The model under review builds one solid part; all positions refer to its coordinate system, in mm. A direction names the side the tool comes from. Coordinates: 2 decimals unless noted, no trailing zeros. Loops run counter-clockwise (first coordinate to the right, second up) from the corner with the lowest first, then second, coordinate; pieces in that order, holes last. Notation, with made-up numbers: M 29,-20 L 81,-20 A21 ccw 81,9 Z; hole C 74.5,48.25 d8. An arc over 180 degrees is marked long. Return JSON: item names as keys, results as strings.
```python
from build123d import *

# Parameters (mm, degrees)
SKETCH1_R           = 2.637642313
SKETCH1_R_2         = 73
BOSS_EXTRUDE1_DEPTH = 20
SKETCH7_R           = 73
SKETCH7_R_2         = 52.25
BOSS_EXTRUDE2_DEPTH = 10
SKETCH8_R           = 73
BOSS_EXTRUDE3_DEPTH = 10
SKETCH9_R           = 11.25
CUT_EXTRUDE1_DEPTH  = 3
SKETCH10_R          = 4.5
CUT_EXTRUDE2_DEPTH  = 89
SKETCH11_R          = 55.2
SKETCH11_R_2        = 52.25
CUT_EXTRUDE3_DEPTH  = 10
SKETCH12_R          = 1
CUT_EXTRUDE4_DEPTH  = 224
SKETCH13_R          = 1
CUT_EXTRUDE5_DEPTH  = 224
SKETCH14_R          = 2.637642313
SKETCH14_R_2        = 1.637642313
BOSS_EXTRUDE4_DEPTH = 20
SKETCH16_R          = 4.637642313
SKETCH16_R_2        = 1.637642313
CUT_EXTRUDE7_DEPTH  = 6
CUT_EXTRUDE11_DEPTH = 15.5
SKETCH19_R          = 6.2
CUT_EXTRUDE12_DEPTH = 144
SKETCH20_R          = 3
SKETCH20_R_2        = 1
CUT_EXTRUDE13_DEPTH = 3.5
SKETCH21_R          = 3
CUT_EXTRUDE14_DEPTH = 3.5
SKETCH22_R          = 3
SKETCH22_R_2        = 1
CUT_EXTRUDE15_DEPTH = 3.5
SKETCH23_R          = 3
CUT_EXTRUDE16_DEPTH = 3.5


with BuildPart() as part:
    # Sketch1 → Boss-Extrude1 (new body)
    with BuildSketch(Plane(origin=(0, 0, 0), x_dir=(1, 0, 0), z_dir=(0, 1, 0))):
        with BuildLine():
            Line((77.460838348, -75.098177713), (77.460838348, 74.577424045))
            ThreePointArc((77.460838348, 74.577424045), (76.578174547, 76.708362964), (74.447235628, 77.591026765))
            Line((74.447235628, 77.591026765), (-75.22836613, 77.591026765))
            ThreePointArc((-75.22836613, 77.591026765), (-77.359305049, 76.708362964), (-78.24196885, 74.577424045))
            Line((-78.24196885, 74.577424045), (-78.24196885, -75.098177713))
            ThreePointArc((-78.24196885, -75.098177713), (-77.359305049, -77.229116632), (-75.22836613, -78.111780433))
            Line((-75.22836613, -78.111780433), (74.447235628, -78.111780433))
            ThreePointArc((74.447235628, -78.111780433), (76.578174547, -77.229116632), (77.460838348, -75.098177713))
        make_face()
        with Locations((-60.604326536, -60.47413812)):
            Circle(SKETCH1_R, mode=Mode.SUBTRACT)
        with Locations((-60.604326536, 59.953384452)):
            Circle(SKETCH1_R, mode=Mode.SUBTRACT)
        with Locations((59.823196035, 59.953384452)):
            Circle(SKETCH1_R, mode=Mode.SUBTRACT)
        with Locations((59.823196035, -60.47413812)):
            Circle(SKETCH1_R, mode=Mode.SUBTRACT)
        with Locations((-0.390565251, -0.260376834)):
            Circle(SKETCH1_R_2, mode=Mode.SUBTRACT)
    extrude(amount=BOSS_EXTRUDE1_DEPTH)

    # Sketch7 → Boss-Extrude2 (add)
    with BuildSketch(Plane(origin=(0, 20, 0), x_dir=(1, 0, 0), z_dir=(0, 1, 0))):
        with Locations((-0.390565251, -0.260376834)):
            Circle(SKETCH7_R)
        with Locations((-0.390565251, -0.260376834)):
            Circle(SKETCH7_R_2, mode=Mode.SUBTRACT)
    extrude(amount=-BOSS_EXTRUDE2_DEPTH)

    # Sketch8 → Boss-Extrude3 (add)
    with BuildSketch(Plane.XZ.offset(-10)):
        with Locations((-0.390565251, 0.260376834)):
            Circle(SKETCH8_R)
    extrude(amount=BOSS_EXTRUDE3_DEPTH)

    # Sketch9 → Cut-Extrude1 (cut)
    with BuildSketch(Plane(origin=(0, 10, 0), x_dir=(1, 0, 0), z_dir=(0, 1, 0))):
        with Locations((-0.390565251, -0.260376834)):
            Circle(SKETCH9_R)
    extrude(amount=-CUT_EXTRUDE1_DEPTH, mode=Mode.SUBTRACT)

    # Sketch10 → Cut-Extrude2 (cut)
    with BuildSketch(Plane(origin=(0, 10, 0), x_dir=(1, 0, 0), z_dir=(0, 1, 0))):
        with Locations((-0.390565251, -0.260376834)):
            Circle(SKETCH10_R)
        with BuildLine():
            ThreePointArc((9.508929686, -11.424371771), (10.773429686, -10.159871771), (9.508929686, -8.895371771))
            ThreePointArc((9.508929686, -8.895371771), (8.244429686, -10.159871771), (9.508929686, -11.424371771))
        make_face()
        with BuildLine():
            ThreePointArc((-10.290060188, -11.424371771), (-9.025560188, -10.159871771), (-10.290060188, -8.895371771))
            ThreePointArc((-10.290060188, -8.895371771), (-11.554560188, -10.159871771), (-10.290060188, -11.424371771))
        make_face()
        with BuildLine():
            ThreePointArc((-10.290060188, 10.903618103), (-11.554560188, 9.639118103), (-10.290060188, 8.374618103))
            ThreePointArc((-10.290060188, 8.374618103), (-9.025560188, 9.639118103), (-10.290060188, 10.903618103))
        make_face()
        with BuildLine():
            ThreePointArc((9.508929686, 10.903618103), (8.244429686, 9.639118103), (9.508929686, 8.374618103))
            ThreePointArc((9.508929686, 8.374618103), (10.773429686, 9.639118103), (9.508929686, 10.903618103))
        make_face()
    extrude(amount=-CUT_EXTRUDE2_DEPTH, mode=Mode.SUBTRACT)

    # Sketch11 → Cut-Extrude3 (cut)
    with BuildSketch(Plane(origin=(0, 20, 0), x_dir=(1, 0, 0), z_dir=(0, 1, 0))):
        with Locations((-0.390565251, -0.260376834)):
            Circle(SKETCH11_R)
        with Locations((-0.390565251, -0.260376834)):
            Circle(SKETCH11_R_2, mode=Mode.SUBTRACT)
    extrude(amount=-CUT_EXTRUDE3_DEPTH, mode=Mode.SUBTRACT)

    # Sketch12 → Cut-Extrude4 (cut)
    with BuildSketch(Plane(origin=(0, 0, -77.591026765), x_dir=(-1, 0, 0), z_dir=(0, 0, -1))):
        with Locations((0.390565251, 15)):
            Circle(SKETCH12_R)
    extrude(amount=-CUT_EXTRUDE4_DEPTH, mode=Mode.SUBTRACT)

    # Sketch13 → Cut-Extrude5 (cut)
    with BuildSketch(Plane.ZY.offset(78.24196885)):
        with Locations((0.260376834, 15)):
            Circle(SKETCH13_R)
    extrude(amount=-CUT_EXTRUDE5_DEPTH, mode=Mode.SUBTRACT)

    # Sketch14 → Boss-Extrude4 (add)
    with BuildSketch(Plane(origin=(0, 20, 0), x_dir=(1, 0, 0), z_dir=(0, 1, 0))):
        with Locations((59.823196035, -60.47413812)):
            Circle(SKETCH14_R)
        with Locations((59.823196035, -60.47413812)):
            Circle(SKETCH14_R_2, mode=Mode.SUBTRACT)
        with Locations((-60.604326536, -60.47413812)):
            Circle(SKETCH14_R)
        with Locations((-60.604326536, -60.47413812)):
            Circle(SKETCH14_R_2, mode=Mode.SUBTRACT)
        with Locations((-60.604326536, 59.953384452)):
            Circle(SKETCH14_R)
        with Locations((-60.604326536, 59.953384452)):
            Circle(SKETCH14_R_2, mode=Mode.SUBTRACT)
        with Locations((59.823196035, 59.953384452)):
            Circle(SKETCH14_R)
        with Locations((59.823196035, 59.953384452)):
            Circle(SKETCH14_R_2, mode=Mode.SUBTRACT)
    extrude(amount=-BOSS_EXTRUDE4_DEPTH)

    # Sketch16 → Cut-Extrude7 (cut)
    with BuildSketch(Plane(origin=(0, 20, 0), x_dir=(1, 0, 0), z_dir=(0, 1, 0))):
        with Locations((59.823196035, -60.47413812)):
            Circle(SKETCH16_R)
        with Locations((59.823196035, -60.47413812)):
            Circle(SKETCH16_R_2, mode=Mode.SUBTRACT)
        with Locations((-60.604326536, -60.47413812)):
            Circle(SKETCH16_R)
        with Locations((-60.604326536, -60.47413812)):
            Circle(SKETCH16_R_2, mode=Mode.SUBTRACT)
        with Locations((-60.604326536, 59.953384452)):
            Circle(SKETCH16_R)
        with Locations((-60.604326536, 59.953384452)):
            Circle(SKETCH16_R_2, mode=Mode.SUBTRACT)
        with Locations((59.823196035, 59.953384452)):
            Circle(SKETCH16_R)
        with Locations((59.823196035, 59.953384452)):
            Circle(SKETCH16_R_2, mode=Mode.SUBTRACT)
    extrude(amount=-CUT_EXTRUDE7_DEPTH, mode=Mode.SUBTRACT)

    # Sketch17 → Cut-Extrude11 (cut)
    with BuildSketch(Plane(origin=(0, 10, 0), x_dir=(1, 0, 0), z_dir=(0, 1, 0))):
        with BuildLine():
            ThreePointArc((42.03584162, 14.549614415), (-0.390565251, 44.549614415), (-42.816972122, 14.549614415))
            Line((-42.816972122, 14.549614415), (-26.371327364, 14.549614415))
            ThreePointArc((-26.371327364, 14.549614415), (-0.390565251, 29.549614415), (25.590196863, 14.549614415))
            Line((25.590196863, 14.549614415), (42.03584162, 14.549614415))
        make_face()
        with BuildLine():
            Line((-26.371327364, -15.450385585), (-42.816972122, -15.450385585))
            ThreePointArc((-42.816972122, -15.450385585), (-0.390565251, -45.450385585), (42.03584162, -15.450385585))
            Line((42.03584162, -15.450385585), (25.590196863, -15.450385585))
            ThreePointArc((25.590196863, -15.450385585), (-0.390565251, -30.450385585), (-26.371327364, -15.450385585))
        make_face()
    extrude(amount=-CUT_EXTRUDE11_DEPTH, mode=Mode.SUBTRACT)

    # Sketch19 → Cut-Extrude12 (cut)
    with BuildSketch(Plane(origin=(0, 10, 0), x_dir=(1, 0, 0), z_dir=(0, 1, 0))):
        with Locations((-36.610454512, -0.450385585)):
            Circle(SKETCH19_R)
    extrude(amount=-CUT_EXTRUDE12_DEPTH, mode=Mode.SUBTRACT)

    # Sketch20 → Cut-Extrude13 (cut)
    with BuildSketch(Plane.ZY.offset(78.24196885)):
        with Locations((0.260376834, 15)):
            Circle(SKETCH20_R)
        with Locations((0.260376834, 15)):
            Circle(SKETCH20_R_2, mode=Mode.SUBTRACT)
    extrude(amount=-CUT_EXTRUDE13_DEPTH, mode=Mode.SUBTRACT)

    # Sketch21 → Cut-Extrude14 (cut)
    with BuildSketch(Plane.XY.offset(78.111780433)):
        with Locations((-0.390565251, 15)):
            Circle(SKETCH21_R)
    extrude(amount=-CUT_EXTRUDE14_DEPTH, mode=Mode.SUBTRACT)

    # Sketch22 → Cut-Extrude15 (cut)
    with BuildSketch(Plane(origin=(77.460838348, 0, 0), x_dir=(0, 0, -1), z_dir=(1, 0, 0))):
        with Locations((-0.260376834, 15)):
            Circle(SKETCH22_R)
        with Locations((-0.260376834, 15)):
            Circle(SKETCH22_R_2, mode=Mode.SUBTRACT)
    extrude(amount=-CUT_EXTRUDE15_DEPTH, mode=Mode.SUBTRACT)

    # Sketch23 → Cut-Extrude16 (cut)
    with BuildSketch(Plane(origin=(0, 0, -77.591026765), x_dir=(-1, 0, 0), z_dir=(0, 0, -1))):
        with Locations((0.390565251, 15)):
            Circle(SKETCH23_R)
    extrude(amount=-CUT_EXTRUDE16_DEPTH, mode=Mode.SUBTRACT)


solid = part.part
```
1. Insertion check: pin 1 Ø5 at (x, y) = (-0.39, 15) entering from -Z; pin 2 Ø7 at (x, z) = (-5, 3) entering from +Y; pin 3 Ø3.5 at (x, z) = (-10.29, -9.64) entering from +Y. Each pin has a flat end and moves straight along its axis. Give the tip position at first contact, or say it passes through.
Check values:
{"pin 1": "z = -74.09", "pin 2": "y = 7", "pin 3": "y = 10"}
2. Add section A-A on z = -42. Give the boundary of the cut face in (x, y).
Check values:
{"outline": "M -78.24,0 L -15.32,0 L -15.32,10 L -35.9,10 L -35.9,20 L -78.24,20 Z; M 14.54,0 L 77.46,0 L 77.46,20 L 35.12,20 L 35.12,10 L 14.54,10 Z"}
3. The part is to be moulded in two halves that separate along X. For faces 1 (the face through (-78.242, 10, -1)), 2 (the face through (-9.318, 8.521, 7.106)), 3 (the face through (-76.52, 12.07, -0.39)), say which applies: released by +X, released by -X, zero draft, split by the parting line, or undercut.
Check values:
{"face 1": "released by -X", "face 2": "undercut", "face 3": "zero draft"}
4. Add section C-C on z = 18. Give the boundary of the cut face in (x, y), plus the area to 3 significant figures.
Check values:
{"outline": "M -78.24,0 L -41.83,0 L -41.83,10 L -52.66,10 L -52.66,20 L -78.24,20 Z; M -24.72,0 L 23.94,0 L 23.94,10 L -24.72,10 Z; M 41.05,0 L 77.46,0 L 77.46,20 L 51.88,20 L 51.88,10 L 41.05,10 Z", "area": "1,730 mm²"}
5. Add section B-B on x = 19. Give the boundary of the cut face in (y, z), plus the area to 3 significant figures.
Check values:
{"outline": "M 0,-77.59 L 20,-77.59 L 20,-51.42 L 10,-51.42 L 10,-40.16 L 0,-40.16 Z; M 0,-22.44 L 10,-22.44 L 10,23.34 L 0,23.34 Z; M 0,41.06 L 10,41.06 L 10,51.94 L 20,51.94 L 20,78.11 L 0,78.11 Z", "area": "1,730 mm²"}
6. Add section D-D on x = -47. Give the boundary of the cut face in (y, z).
Check values:
{"outline": "M 0,-77.59 L 20,-77.59 L 20,-29.31 L 10,-29.31 L 10,29.83 L 20,29.83 L 20,78.11 L 0,78.11 Z"}
7. To check wall thickness, follow line 1 (X direction, y = 7.25, z = 15.5); line 2 (X direction, y = 2, z = 9.5); line 3 (Z direction, x = -34.5, y = 7). State the ranges of each line that lie inside material, in increasing order.
Check values:
{"line 1": "-78.24 to -42.8, -26.34 to 25.56, 42.02 to 77.46", "line 2": "-78.24 to -11.37, -9.21 to 8.43, 10.59 to 77.46", "line 3": "-77.59 to -28.9, -14.55 to -5.38, 6.28 to 15.45, 29.8 to 78.11"}
8. Machinability: for faces 4 (the face through (73.961, 16, 1)), 5 (the face through (-1, 16, 74.612)), 6 (the face through (34, 5, 15.45)), 7 (the face through (-0.3, 13.7, -74.091)), 8 (the face through (-41.075, 15.07, -37.046)), which of the approach directions +Z, -Z, +X, -X, +Y, -Y give a long, thin tool a straight path to every point of the face, cutting with its end or side? Answer none if there is none.
Check values:
{"face 4": "+X", "face 5": "+Z", "face 6": "+Y, -Y", "face 7": "-Z", "face 8": "+Y"}
